Autodesk Inventor part; units mm, degrees
ref_plane "YZ Plane" through (0, 0, 0) normal (1, 0, 0) x (0, 1, 0)
ref_plane "XZ Plane" through (0, 0, 0) normal (0, 1, 0) x (-1, 0, 0)
ref_plane "XY Plane" through (0, 0, 0) normal (0, 0, 1) x (1, 0, 0)
sketch "Sketch1" plane through (0, 0, 0) normal (0, 0, 1) x (1, 0, 0)
  line L0 (-15, 0.5) -> (15, 0.5)
  line L1 (15, 0.5) -> (15, -0.5)
  line L2 (15, -0.5) -> (-15, -0.5)
  line L3 (-15, -0.5) -> (-15, 0.5)
  line L4 (-15, 0.5) -> (15, -0.5) construction
  line L5 (15, 0.5) -> (-15, -0.5) construction
  line L6 (-14, 10.4333) -> (-13, 10.4333)
  line L7 (-13, 10.4333) -> (-13, 0.4333)
  line L8 (-13, 0.4333) -> (-14, 0.4333)
  line L9 (-14, 0.4333) -> (-14, 10.4333)
  line L10 (-14, 10.4333) -> (-13, 0.4333) construction
  line L11 (-13, 10.4333) -> (-14, 0.4333) construction
  line L12 (-11, 10.4333) -> (-10, 10.4333)
  line L13 (-10, 10.4333) -> (-10, 0.4333)
  line L14 (-10, 0.4333) -> (-11, 0.4333)
  line L15 (-11, 0.4333) -> (-11, 10.4333)
  line L16 (-11, 10.4333) -> (-10, 0.4333) construction
  line L17 (-10, 10.4333) -> (-11, 0.4333) construction
  line L18 (-8, 10.4333) -> (-7, 10.4333)
  line L19 (-7, 10.4333) -> (-7, 0.4333)
  line L20 (-7, 0.4333) -> (-8, 0.4333)
  line L21 (-8, 0.4333) -> (-8, 10.4333)
  line L22 (-8, 10.4333) -> (-7, 0.4333) construction
  line L23 (-7, 10.4333) -> (-8, 0.4333) construction
  line L24 (-5, 10.4333) -> (-4, 10.4333)
  line L25 (-4, 10.4333) -> (-4, 0.4333)
  line L26 (-4, 0.4333) -> (-5, 0.4333)
  line L27 (-5, 0.4333) -> (-5, 10.4333)
  line L28 (-5, 10.4333) -> (-4, 0.4333) construction
  line L29 (-4, 10.4333) -> (-5, 0.4333) construction
  line L30 (-2, 10.4333) -> (-1, 10.4333)
  line L31 (-1, 10.4333) -> (-1, 0.4333)
  line L32 (-1, 0.4333) -> (-2, 0.4333)
  line L33 (-2, 0.4333) -> (-2, 10.4333)
  line L34 (-2, 10.4333) -> (-1, 0.4333) construction
  line L35 (-1, 10.4333) -> (-2, 0.4333) construction
  line L36 (1, 10.4333) -> (2, 10.4333)
  line L37 (2, 10.4333) -> (2, 0.4333)
  line L38 (2, 0.4333) -> (1, 0.4333)
  line L39 (1, 0.4333) -> (1, 10.4333)
  line L40 (1, 10.4333) -> (2, 0.4333) construction
  line L41 (2, 10.4333) -> (1, 0.4333) construction
  line L42 (4, 10.4333) -> (5, 10.4333)
  line L43 (5, 10.4333) -> (5, 0.4333)
  line L44 (5, 0.4333) -> (4, 0.4333)
  line L45 (4, 0.4333) -> (4, 10.4333)
  line L46 (4, 10.4333) -> (5, 0.4333) construction
  line L47 (5, 10.4333) -> (4, 0.4333) construction
  line L48 (7, 10.4333) -> (8, 10.4333)
  line L49 (8, 10.4333) -> (8, 0.4333)
  line L50 (8, 0.4333) -> (7, 0.4333)
  line L51 (7, 0.4333) -> (7, 10.4333)
  line L52 (7, 10.4333) -> (8, 0.4333) construction
  line L53 (8, 10.4333) -> (7, 0.4333) construction
  line L54 (10, 10.4333) -> (11, 10.4333)
  line L55 (11, 10.4333) -> (11, 0.4333)
  line L56 (11, 0.4333) -> (10, 0.4333)
  line L57 (10, 0.4333) -> (10, 10.4333)
  line L58 (10, 10.4333) -> (11, 0.4333) construction
  line L59 (11, 10.4333) -> (10, 0.4333) construction
  line L60 (13, 10.4333) -> (14, 10.4333)
  line L61 (14, 10.4333) -> (14, 0.4333)
  line L62 (14, 0.4333) -> (13, 0.4333)
  line L63 (13, 0.4333) -> (13, 10.4333)
  line L64 (13, 10.4333) -> (14, 0.4333) construction
  line L65 (14, 10.4333) -> (13, 0.4333) construction
  point P0 (0, 0)
  point P1 (-13.5, 5.4333)
  point P2 (-12, 0.5)
  point P3 (-10.5, 5.4333)
  point P4 (-9, 0.5)
  point P5 (-7.5, 5.4333)
  point P6 (-6, 0.5)
  point P7 (-4.5, 5.4333)
  point P8 (-3, 0.5)
  point P9 (-1.5, 5.4333)
  point P10 (0, 0.5)
  point P11 (1.5, 5.4333)
  point P12 (3, 0.5)
  point P13 (4.5, 5.4333)
  point P14 (6, 0.5)
  point P15 (7.5, 5.4333)
  point P16 (9, 0.5)
  point P17 (10.5, 5.4333)
  point P18 (12, 0.5)
  point P19 (13.5, 5.4333)
  point P20 (13, 0.5)
  point P21 (11, 0.5)
  point P22 (10, 0.5)
  point P23 (8, 0.5)
  point P24 (7, 0.5)
  point P25 (5, 0.5)
  point P26 (4, 0.5)
  point P27 (2, 0.5)
  point P28 (1, 0.5)
  point P29 (-1, 0.5)
  point P30 (-2, 0.5)
  point P31 (-4, 0.5)
  point P32 (-5, 0.5)
  point P33 (-7, 0.5)
  point P34 (-8, 0.5)
  point P35 (-10, 0.5)
  point P36 (-11, 0.5)
  point P37 (-13, 0.5)
  point P38 (14, 0.5)
  point P39 (-14, 0.5)
  dimension "d0" = 1
  dimension "d1" = 30
  dimension "d2" = 1
  dimension "d3" = 10
  dimension "d6" = 3
  dimension "d13" = 1
  dimension "d14" = 1
extrude "Extrusion1" add sketch "Sketch1" along normal blind 30
properties part number "cooler_plate" material "Aluminum 6061"
Here's how the part is built. I have some questions about the finished solid (model axes, mm). A direction names the side the tool comes from. Give positions to 0.01 mm unless a question says otherwise; leave off trailing zeros. Loops run counter-clockwise (first coordinate to the right, second up) from the corner with the lowest first, then second, coordinate; pieces in that order, holes last. Notation, with made-up numbers: M 63,-24 L 75,-24 A22 ccw 75,15 Z; hole C 27,8 d2. An arc over 180 degrees is marked long. Return JSON: item names as keys, results as strings.
Item 1: I'm going to push flat-ended pins straight in: pin 1 Ø1.5 at (y, z) = (4, 12.5) entering from +X; pin 2 Ø0.6 at (x, z) = (12, 15.5) entering from +Y; pin 3 Ø5 at (y, z) = (6, 16.5) entering from -X. Where does each tip first touch, or does it pass through?
A:
{"pin 1": "stops at x = 14", "pin 2": "stops at y = 0.5", "pin 3": "stops at x = -14"}
Item 2: On a 3-axis mill with a long thin cutter (end or side, diameter ignored), from which of +Z, -Z, +X, -X, +Y, -Y can I reach the whole of each face in a straight line? I mean faces 4 (the flat face through (-15, 0, 15)), 5 (the flat face through (13.5, 10.433, 14.8)), 6 (the flat face through (-2, 5, 15)), 7 (the flat face through (-14, 5, 15)), 8 (the flat face through (14, 6, 15)). Say none if no direction works.
A:
{"face 4": "+Z, -Z, -X, +Y, -Y", "face 5": "+Z, -Z, +X, -X, +Y", "face 6": "+Z, -Z, +Y", "face 7": "+Z, -Z, -X, +Y", "face 8": "+Z, -Z, +X, +Y"}
Item 3: Please list where this line runs through material, in increasing order: line 1 (Y direction, x = -3.5, z = 9.25).
A:
{"line 1": "y = -0.5 to 0.5"}
Item 4: Imagine slicing it at A-A on y = 2.75. State how many separate pieces and enclosed holes the cut face has, then the cut area to 3 significant figures.
A:
{"separate pieces": "10", "enclosed holes": "0", "area": "300 mm^2"}
Item 5: Imagine slicing it at B-B on x = -8.75. List the corners of the cut face in (y, z) for me.
A:
{"outline": "M -0.5,0 L 0.5,0 L 0.5,30 L -0.5,30 Z"}
Item 6: Thinking about a two-plate mould opening in X: for faces 1 (the flat face through (-13, 6, 15)), 2 (the flat face through (15, 0, 15)), 3 (the flat face through (-14.5, 0.5, 14.8)), which applies, released by +X, released by -X, zero draft, split by the parting line, or undercut?
A:
{"face 1": "undercut", "face 2": "released by +X", "face 3": "zero draft"}
